from build123d import *

# Parameters (mm, degrees)
F0_W      = 212
F0_H      = 160
F1_DEPTH  = 5
F2_W      = 152
F2_H      = 80
F3_DEPTH  = 80
F4_R      = 6
F5_DEPTH  = 16
F6_R      = 6
F7_DEPTH  = 16
F9_D      = 8.8
F9_DEPTH  = 15
F9_TIP    = 2.6437867237
F10_R     = 20
F11_R     = 17.5
F11_R_2   = 6
F12_DEPTH = 10
F13_W     = 28
F13_H     = 50
F14_DEPTH = 4
F16_D     = 9
F16_DEPTH = 15
F16_TIP   = 2.7038727856


with BuildPart() as f1:
    # F0 (on Top) → F1 (new body)
    with BuildSketch(Plane.XY):
        Rectangle(F0_W, F0_H)
    extrude(amount=F1_DEPTH)

    # F2 (on face) → F3 (join)
    with BuildSketch(Plane.XY.offset(5)):
        with Locations((0, 25)):
            Rectangle(F2_W, F2_H)
    extrude(amount=F3_DEPTH)

    # F4 (on face) → F5 (join)
    with BuildSketch(Plane.XZ.offset(15)):
        with Locations((-36, 45)):
            Circle(F4_R)
    extrude(amount=F5_DEPTH)

    # F6 (on face) → F7 (join)
    with BuildSketch(Plane(origin=(0, 65, 0), x_dir=(-1, 0, 0), z_dir=(0, 1, 0))):
        with Locations((-36, 45)):
            Circle(F6_R)
    extrude(amount=F7_DEPTH)

    # F9
    with Locations(Plane(origin=(0, 81, 0), x_dir=(-1, 0, 0), z_dir=(0, 1, 0))):
        with Locations((-36, 45)):
            Hole(F9_D / 2, depth=F9_DEPTH)
            with Locations((0, 0, -(F9_DEPTH + F9_TIP / 2))):  # 118° drill point
                Cone(0, F9_D / 2, F9_TIP, mode=Mode.SUBTRACT)

    # F10
    f10_edges = [f1.edges().sort_by_distance(p)[0] for p in [
        (106, -80, 2.5),
        (106, 80, 2.5),
        (-106, 80, 2.5),
        (-106, -80, 2.5),
    ]]
    fillet(f10_edges, radius=F10_R)

    # F11 (on face) → F12 (join)
    with BuildSketch(Plane(origin=(0, 65, 0), x_dir=(-1, 0, 0), z_dir=(0, 1, 0))):
        with Locations((-36, 45)):
            Circle(F11_R)
        with Locations((-36, 45)):
            Circle(F11_R_2, mode=Mode.SUBTRACT)
    extrude(amount=F12_DEPTH)

    # F13 (on face) → F14 (join)
    with BuildSketch(Plane.XY.offset(5)):
        with Locations((-90, 25)):
            Rectangle(F13_W, F13_H)
        with Locations((90, 25)):
            Rectangle(F13_W, F13_H)
    extrude(amount=F14_DEPTH)

    # F16
    with Locations(Plane.XY.offset(9)):
        with Locations((-94, 25), (94, 25)):
            Hole(F16_D / 2, depth=F16_DEPTH)
            with Locations((0, 0, -(F16_DEPTH + F16_TIP / 2))):  # 118° drill point
                Cone(0, F16_D / 2, F16_TIP, mode=Mode.SUBTRACT)


solid = f1.part
Geometry check sheet. Reference: the model listing, model coordinates, mm. A direction names the side the tool comes from. Round coordinates to 2 decimals unless told otherwise and drop trailing zeros. Loops run counter-clockwise (first coordinate to the right, second up) from the corner with the lowest first, then second, coordinate; pieces in that order, holes last. Notation, with made-up numbers: (0.25, -13) - (9.25, -13) arc R14 ccw to (9.25, -4) - close; hole circle Ø11 at (-37, 57.25). An arc over 180 degrees is marked (long way). One line per question, with ' | ' between items. Start each with the question number.
1. Cross-section at A-A on y = 25. Record the cut outline in (x, z).
2. Cross-section at B-B on y = -26. Record the cut outline in (x, z), then the cut area to 3 significant figures.
3. Cross-section at D-D on x = -94. Record the cut outline in (y, z), then the cut area to 3 significant figures.
4. Scan lines: line 1 (Z direction, x = 36, y = 73.25); line 2 (Y direction, x = 94, z = 7.25); line 3 (Y direction, x = -78, z = 6). Record each from-to range of solid material in increasing order. Write a range as [from, to].
5. Draft check along X on faces 1 (the face through (-1, 80, 2)), 2 (the face through (-89.504, 25.198, 4.437)), 3 (the face through (42, 78, 45)). Enter one of: released by +X, released by -X, zero draft, split by the parting line, or undercut.
6. Cross-section at C-C on x = -36. Record the cut outline in (y, z).
7. Depth check by flat-ended pin: pin 1 (2 mm diameter, centred on x = 84, z = 7.5, fed in from -Y); pin 2 (4 mm diameter, centred on y = 29, z = 45.5, fed in from -X); pin 3 (5.5 mm diameter, centred on x = 36, z = 45, fed in from +Y). Enter the tip coordinate at first touch or a pass-through.
8. Tool access check on faces 4 (the face through (-87, 25, 9)), 5 (the face through (38.03, 73.395, 41.096)), 6 (the face through (-100.297, -73.986, 2.535)), 7 (the face through (-42, -23, 45)), 8 (the face through (87, 25, 9)). Record the directions out of +Z, -Z, +X, -X, +Y, -Y that give a thin tool (end or side, any length) a straight path to the whole face; none if there is none.
Taken from the geometry:
1) outline: (-106, 0) - (-98.5, 0) - (-98.5, 9) - (-104, 9) - (-104, 5) - (-106, 5) - close; (-89.5, 0) - (89.5, 0) - (89.5, 9) - (76, 9) - (76, 85) - (-76, 85) - (-76, 9) - (-89.5, 9) - close; (98.5, 0) - (106, 0) - (106, 5) - (104, 5) - (104, 9) - (98.5, 9) - close
2) outline: (-106, 0) - (106, 0) - (106, 5) - (-106, 5) - close; circle Ø12 at (-36, 45) | area: 1,170 mm²
3) outline: (-78.33, 0) - (20.5, 0) - (20.5, 9) - (0, 9) - (0, 5) - (-78.33, 5) - close; (29.5, 0) - (78.33, 0) - (78.33, 5) - (50, 5) - (50, 9) - (29.5, 9) - close | area: 902 mm²
4) line 1: [0, 5], [27.5, 40.6], [49.4, 62.5] | line 2: [0, 20.5], [29.5, 50] | line 3: [0, 50]
5) face 1: zero draft | face 2: undercut | face 3: split by the parting line
6) outline: (-80, 0) - (80, 0) - (80, 5) - (65, 5) - (65, 85) - (-15, 85) - (-15, 51) - (-31, 51) - (-31, 39) - (-15, 39) - (-15, 5) - (-80, 5) - close
7) pin 1: y = 0 | pin 2: x = -76 | pin 3: y = 65.01
8) face 4: +Z, -X, +Y, -Y | face 5: +Y | face 6: +Z, -Z, -X, -Y | face 7: -Y | face 8: +Z, +X, +Y, -Y
